from build123d import *

# Parameters (mm, degrees)
F0_W        = 127
F0_H        = 76.2
F0_R        = 5.2244265331
F0_R_2      = 6.35
F1_DEPTH    = 50.8
F2_R        = 15.1393609574
F3_DEPTH    = 138.938
F4_T1_DEPTH = 116.1207478943
F4_T3_DEPTH = 192.3207478943
F5_R        = 12.7


# Not quite as in the source:
# - a fillet or chamfer that OpenCascade refuses, or shapes differently, is made with other operations: its cross-section is extruded or revolved along the edge and cut away or added


with BuildPart() as f1:
    # F0 (on Front) → F1 (new body)
    with BuildSketch(Plane.XZ):
        with Locations((-1.653669402, -66.8124542732)):
            Rectangle(F0_W, F0_H)
        with Locations((-30.8793820441, -68.7773153186)):
            Circle(F0_R, mode=Mode.SUBTRACT)
        with Locations((42.796330598, -54.1124542732)):
            Circle(F0_R_2, mode=Mode.SUBTRACT)
    extrude(amount=F1_DEPTH)

    # F2 (on face) → F3 (cut)
    with BuildSketch(Plane.XZ.offset(50.8)):
        with Locations((26.5990737826, -85.8985558152)):
            Circle(F2_R)
    extrude(amount=-F3_DEPTH, mode=Mode.SUBTRACT)

    # F4: chamfer of 12.7 on 4 edges, made by hand

    # F4_s2 → F4_t1 (cut)
    with BuildSketch(Plane.XZ.offset(-32.6603739472)):
        Polygon((61.846330598, -92.2124542732), (49.146330598, -104.9124542732), (61.846330598, -104.9124542732), align=None)
        Polygon((-65.153669402, -92.2124542732), (-52.453669402, -104.9124542732), (-65.153669402, -104.9124542732), align=None)
    extrude(amount=F4_T1_DEPTH, mode=Mode.SUBTRACT)

    # F4_s4 → F4_t3 (cut)
    with BuildSketch(Plane.YZ.offset(-97.8140433492)):
        Polygon((-50.8, -92.2124542732), (-38.1, -104.9124542732), (-50.8, -104.9124542732), align=None)
        Polygon((0, -92.2124542732), (-12.7, -104.9124542732), (0, -104.9124542732), align=None)
    extrude(amount=F4_T3_DEPTH, mode=Mode.SUBTRACT)

    # F5
    f5_edges = [f1.edges().sort_by_distance(p)[0] for p in [
        (-1.653669, -38.1, -104.912454),
        (-1.653669, -12.7, -104.912454),
        (49.146331, -25.4, -104.912454),
        (-52.453669, -25.4, -104.912454),
    ]]
    fillet(f5_edges, radius=F5_R)


solid = f1.part
Could you check a few things on this model? Use its own coordinates, in mm. Give positions to 0.01 mm unless a question says otherwise; leave off trailing zeros. Loops run counter-clockwise (first coordinate to the right, second up) from the corner with the lowest first, then second, coordinate; pieces in that order, holes last. Notation, with made-up numbers: (32.5, -30) -> (61.5, -30) arc R21 cw to (61.5, 6) -> close; hole circle Ø1 at (43.5, 65.5). An arc over 180 degrees is marked (long way). Answer as CSV lines item,"result". Start each with the question number.
(1) If we section it at A-A on y = -38: Write out the boundary of the cut face in (x, z), then the cut area to 3 significant figures.
(2) I'm going to push flat-ended pins straight in: pin 1 Ø1 at (x, y) = (-27.5, -40.5) entering from -Z; pin 2 Ø3 at (x, y) = (-28, -8) entering from -Z; pin 3 Ø9.5 at (x, z) = (-30.88, -68.78) entering from +Y; pin 4 Ø1.5 at (y, z) = (-12.5, -96) entering from +X. Where does each tip first touch, or does it pass through?
(3) If we section it at C-C on x = 16.5: Write out the boundary of the cut face in (y, z), then the cut area to 3 significant figures.
(4) If we section it at D-D on x = 54.5: Write out the boundary of the cut face in (y, z).
(5) We'd pull the mould along X, two halves only. Please class faces 1 (the flat face through (61.846, -25, -61)), 2 (the cylindrical face through (-31.559, -25.044, -63.597)), 3 (the flat face through (-2.54, -4.43, -96.64)): released by +X, released by -X, zero draft, split by the parting line, or undercut.
(6) I need wall thicknesses on probe 1 along X at (y, z) = (-13, -72); probe 2 along Z at (x, y) = (5.5, -44); probe 3 along Z at (x, y) = (38, -2). Which ranges of each line are inside material? Lowest first, please.
(7) If we section it at B-B on z = -76: Write out the boundary of the cut face in (x, y), then the cut area to 3 significant figures.
Computed:
1,outline,"(-65.15, -92.21) -> (-56.17, -101.19) arc R12.7 ccw to (-52.35, -103.82) -> (49.05, -103.82) arc R12.7 ccw to (52.87, -101.19) -> (61.85, -92.21) -> (61.85, -28.71) -> (-65.15, -28.71) -> close; hole circle Ø10.45 at (-30.88, -68.78); hole circle Ø30.28 at (26.6, -85.9); hole circle Ø12.7 at (42.8, -54.11)"
1,area,"8,470 mm2"
2,pin 1,"stops at z = -102.7"
2,pin 2,"stops at z = -101.68"
2,pin 3,"passes through"
2,pin 4,"stops at x = 58.81"
3,outline,"(-50.8, -74.62) -> (0, -74.62) -> (0, -28.71) -> (-50.8, -28.71) -> close; (-45.84, -97.18) -> (-41.82, -101.19) arc R12.7 ccw to (-32.84, -104.91) -> (-17.96, -104.91) arc R12.7 ccw to (-8.98, -101.19) -> (-4.96, -97.18) -> close"
3,area,"2,580 mm2"
4,outline,"(-50.8, -92.21) -> (-43.45, -99.56) -> (-7.35, -99.56) -> (0, -92.21) -> (0, -28.71) -> (-50.8, -28.71) -> close"
5,face 1,"released by +X"
5,face 2,"undercut"
5,face 3,"zero draft"
6,probe 1,"x = -65.15 to -34.99, -26.77 to 20.6, 32.6 to 61.85"
6,probe 2,"z = -99.01 to -28.71"
6,probe 3,"z = -75.94 to -58.27, -49.95 to -28.71"
7,outline,"(-65.15, -50.8) -> (15.14, -50.8) -> (15.14, 0) -> (-65.15, 0) -> close; (38.05, -50.8) -> (61.85, -50.8) -> (61.85, 0) -> (38.05, 0) -> close"
7,area,"5,290 mm2"
